Here's how the part is built. I have some questions about the finished solid (model axes, mm). A direction names the side the tool comes from. Coordinates: 2 decimals unless noted, no trailing zeros. Write each loop counter-clockwise with the first axis right and the second up, starting at its lowest first coordinate (ties: lowest second). Pieces come first, ordered by that corner, then holes. Notation, with made-up numbers: (-38.5, 20) -> (-0.5, 20) arc R27 cw to (-0.5, 50) -> close; hole circle Ø2 at (-28, 23). An arc over 180 degrees is marked (long way). Put each result on its own line as item: value.
```python
from build123d import *

# Parameters (mm, degrees)
SKETCH_2_W             = 110
SKETCH_2_H             = 50
SM_BASE_FLANGE_1_DEPTH = 3
OTHER_START            = -25
OTHER_1_DEPTH          = 50
OTHER_1_2_DEPTH        = 50
SKETCH_8_R             = 2
CUT_EXTRUDE_1_DEPTH    = 10
FILLET_1_R             = 3
SKETCH_9_R             = 13
CUT_EXTRUDE_2_DEPTH    = 10
SKETCH_10_R            = 1.65
CUT_EXTRUDE_3_DEPTH    = 82.01751709


# Read off the part's stored shape, not the designer's step: 绘制的折弯1
# Sheet-metal steps are written as plain solids
with BuildPart() as part:
    # Sketch 2 → 基体-法兰1 (new body)
    with BuildSketch(Plane.XY):
        Rectangle(SKETCH_2_W, SKETCH_2_H)
    extrude(amount=-SM_BASE_FLANGE_1_DEPTH)

    # Other 1 outline → Other 1 (cut)
    with BuildSketch(Plane(origin=(0, 0, 0), x_dir=(1, 0, 0), z_dir=(0, 1, 0)).offset(OTHER_START)):
        with BuildLine():
            ThreePointArc((-1.756621532, 3), (0.610845469, 2.154295979), (1.906655689, 0))
            Line((1.906655689, 0), (55, 0))
            Line((55, 0), (55, 3))
            Line((55, 3), (-1.756621532, 3))
        make_face()
    extrude(amount=OTHER_1_DEPTH, mode=Mode.SUBTRACT)

    # Other 1 2 outline → Other 1 2 (add)
    with BuildSketch(Plane(origin=(0, 0, 0), x_dir=(1, 0, 0), z_dir=(0, 1, 0)).offset(OTHER_START)):
        with BuildLine():
            Line((-1.020021532, -0.7366), (-1.020021532, -53.979978468))
            Line((-1.020021532, -53.979978468), (1.979978468, -53.979978468))
            Line((1.979978468, -53.979978468), (1.979978468, -0.7366))
            ThreePointArc((1.979978468, -0.7366), (1.961602589, -0.36647982), (1.906655689, 0))
            Line((1.906655689, 0), (-1.756621532, 0))
            ThreePointArc((-1.756621532, 0), (-1.235766677, -0.215745145), (-1.020021532, -0.7366))
        make_face()
    extrude(amount=OTHER_1_2_DEPTH)

    # 草图8 → 切除-拉伸1 (cut)
    with BuildSketch(Plane.ZY.offset(1.020021532)):
        with Locations((12, 0)):
            Circle(SKETCH_8_R)
        with Locations((42, 0)):
            Circle(SKETCH_8_R)
        with Locations((27, 15)):
            Circle(SKETCH_8_R)
        with Locations((27, -15)):
            Circle(SKETCH_8_R)
    extrude(amount=-CUT_EXTRUDE_1_DEPTH, mode=Mode.SUBTRACT)

    # 圆角1
    fillet_1_edges = [part.edges().sort_by_distance(p)[0] for p in [
        (-55, -25, -1.5),
        (-55, 25, -1.5),
        (0.479978468, -25, 53.979978468),
        (0.479978468, 25, 53.979978468),
    ]]
    fillet(fillet_1_edges, radius=FILLET_1_R)

    # 草图9 → 切除-拉伸2 (cut)
    with BuildSketch(Plane.XY):
        with Locations((-33, 0)):
            Circle(SKETCH_9_R)
    extrude(amount=-CUT_EXTRUDE_2_DEPTH, mode=Mode.SUBTRACT)

    # 草图10 → 切除-拉伸3 (cut, through all)
    with BuildSketch(Plane.XY):
        with Locations((-20.625631329, 12.374368671)):
            Circle(SKETCH_10_R)
        with Locations((-20.625631329, -12.374368671)):
            Circle(SKETCH_10_R)
        with Locations((-45.374368671, -12.374368671)):
            Circle(SKETCH_10_R)
        with Locations((-45.374368671, 12.374368671)):
            Circle(SKETCH_10_R)
    extrude(amount=-CUT_EXTRUDE_3_DEPTH, mode=Mode.SUBTRACT)


solid = part.part
```
Item 1: Imagine slicing it at A-A on z = 12. Write out the boundary of the cut face in (x, y), then the cut area to 3 significant figures.
Output:
outline: (-1.02, -25) -> (1.98, -25) -> (1.98, -2) -> (-1.02, -2) -> close; (-1.02, 2) -> (1.98, 2) -> (1.98, 25) -> (-1.02, 25) -> close
area: 138 mm²
Item 2: Imagine slicing it at D-D on z = 27. Write out the boundary of the cut face in (x, y).
Output:
outline: (-1.02, -25) -> (1.98, -25) -> (1.98, -17) -> (-1.02, -17) -> close; (-1.02, -13) -> (1.98, -13) -> (1.98, 13) -> (-1.02, 13) -> close; (-1.02, 17) -> (1.98, 17) -> (1.98, 25) -> (-1.02, 25) -> close
Item 3: Which directions (+Z, -Z, +X, -X, +Y, -Y) give clear straight access to the entire face, cutting with the end or side of a thin tool? Please do faces 4 (the cylindrical face through (-54.1, -24.14, -1.52)), 5 (the flat face through (-17, 0, 0)).
Output:
face 4: +Z, -Z, -X, -Y
face 5: +Z, -X, +Y, -Y
Item 4: If we mould it in two halves opening along X, with no side actions, what happens to faces 1 (the cylindrical face through (0, 0, 40)), 2 (the cylindrical face through (-47.023, 12.447, -1.479)), 3 (the flat face through (-1.02, 0, 27))? For each: released by +X, released by -X, zero draft, split by the parting line, or undercut.
Output:
face 1: zero draft
face 2: undercut
face 3: released by -X
Item 5: Please list where these lines run through material, in increasing order: line 1 along Y through (x, z) = (-0.15, 27); line 2 along Y through (x, z) = (0, 12); line 3 along X through (y, z) = (-15, 4). Write a range as from..to.
Output:
line 1: y = -25..-17, -13..13, 17..25
line 2: y = -25..-2, 2..25
line 3: x = -1.02..1.98
Item 6: For P1, Ø5.5, axis at x = -45.37, y = -12.37, coming from the +Z side; P2, Ø10, axis at y = -3, z = 42.5, coming from the -X side, each with a flat end and sliding along its axis, tell me the tip position at first contact or that it passes through.
Output:
P1: stops at z = 0
P2: stops at x = -1.02
Item 7: Imagine slicing it at B-B on y = -15. Write out the boundary of the cut face in (x, z), then the cut area to 3 significant figures.
Output:
outline: (-55, -3) -> (-1.76, -3) arc R3.74 ccw to (1.98, 0.74) -> (1.98, 25) -> (-1.02, 25) -> (-1.02, 0.74) arc R0.74 cw to (-1.76, 0) -> (-55, 0) -> close; (-1.02, 29) -> (1.98, 29) -> (1.98, 53.98) -> (-1.02, 53.98) -> close
area: 318 mm²
Item 8: Imagine slicing it at C-C on x = -24.5. Write out the boundary of the cut face in (y, z).
Output:
outline: (-25, -3) -> (-9.84, -3) -> (-9.84, 0) -> (-25, 0) -> close; (9.84, -3) -> (25, -3) -> (25, 0) -> (9.84, 0) -> close
